Part model, mm, in its own coordinate system. A direction names the side the tool comes from. Coordinates: 2 decimals unless noted, no trailing zeros. Loops run counter-clockwise (first coordinate to the right, second up) from the corner with the lowest first, then second, coordinate; pieces in that order, holes last.
```python
from build123d import *

# Parameters (mm, degrees)
SKETCH1_R           = 7.9375
BOSS_EXTRUDE1_DEPTH = 27.2415
SKETCH2_R           = 2.4765
CUT_EXTRUDE1_DEPTH  = 49.665241675
CUT_EXTRUDE2_DEPTH  = 49.665241675
SKETCH4_R           = 7.9375
CUT_EXTRUDE3_DEPTH  = 41.615884673
FILLET1_R           = 6.35
FILLET2_R           = 3.175
FILLET3_R           = 12.7
FILLET4_R           = 2.54
FILLET5_R           = 2.54


with BuildPart() as part:
    # Sketch1 → Boss-Extrude1 (new, symmetric)
    with BuildSketch(Plane.XY):
        with BuildLine():
            Line((11.25771962, 2.316093955), (14.0335, -11.176))
            Line((14.0335, -11.176), (14.0335, -28.956))
            Line((14.0335, -28.956), (11.2014, -28.956))
            Line((11.2014, -28.956), (11.2014, -15.1638))
            Line((11.2014, -15.1638), (-11.2014, -15.1638))
            Line((-11.2014, -15.1638), (-11.2014, -28.956))
            Line((-11.2014, -28.956), (-14.0335, -28.956))
            Line((-14.0335, -28.956), (-14.0335, -11.176))
            Line((-14.0335, -11.176), (-11.25771962, 2.316093955))
            ThreePointArc((-11.25771962, 2.316093955), (0, 11.4935), (11.25771962, 2.316093955))
        make_face()
        Circle(SKETCH1_R, mode=Mode.SUBTRACT)
    extrude(amount=BOSS_EXTRUDE1_DEPTH, both=True)

    # Sketch2 → Cut-Extrude1 (cut, through all)
    with BuildSketch(Plane(origin=(14.0335, 0, 0), x_dir=(0, 0, -1), z_dir=(1, 0, 0))):
        with Locations(Location((-20.066, -22.7838, 0), (0, 0, 90))):
            Circle(SKETCH2_R)
        with Locations(Location((-12.7, -22.7838, 0), (0, 0, 90))):
            Circle(SKETCH2_R)
        with Locations(Location((-5.334, -22.7838, 0), (0, 0, 90))):
            Circle(SKETCH2_R)
        with Locations(Location((5.334, -22.7838, 0), (0, 0, 90))):
            Circle(SKETCH2_R)
        with Locations(Location((12.7, -22.7838, 0), (0, 0, 90))):
            Circle(SKETCH2_R)
        with Locations(Location((20.066, -22.7838, 0), (0, 0, 90))):
            Circle(SKETCH2_R)
    extrude(amount=-CUT_EXTRUDE1_DEPTH, mode=Mode.SUBTRACT)

    # Sketch3 → Cut-Extrude2 (cut, through all)
    with BuildSketch(Plane(origin=(14.0335, 0, 0), x_dir=(0, 0, -1), z_dir=(1, 0, 0))):
        Polygon((14.7955, -12.573), (-14.7955, -12.573), (-14.7955, -2.413), (-21.6535, 7.38123903), (-21.6535, 11.4935), (21.6535, 11.4935), (21.6535, 7.38123903), (14.7955, -2.413), align=None)
    extrude(amount=-CUT_EXTRUDE2_DEPTH, mode=Mode.SUBTRACT)

    # Sketch4 → Cut-Extrude3 (cut, through all)
    with BuildSketch(Plane.XZ.offset(15.1638)):
        Circle(SKETCH4_R)
    extrude(amount=-CUT_EXTRUDE3_DEPTH, mode=Mode.SUBTRACT)

    # Fillet1
    fillet1_edges = [part.edges().sort_by_distance(p)[0] for p in [
        (12.61745, -28.956, -27.2415),
        (-12.61745, -28.956, -27.2415),
        (-12.61745, -28.956, 27.2415),
        (12.61745, -28.956, 27.2415),
    ]]
    fillet(fillet1_edges, radius=FILLET1_R)

    # Fillet2
    fillet2_edges = [part.edges().sort_by_distance(p)[0] for p in [
        (0, -12.573, 14.7955),
        (0, -12.573, -14.7955),
    ]]
    fillet(fillet2_edges, radius=FILLET2_R)

    # Fillet3
    # the kernel refuses this fillet: 12.7 mm, written as the material it adds along each edge
    with BuildSketch(Plane(origin=(18.820836014, 7.38123903, 21.6535), x_dir=(0, -0.8191520442889931, -0.5735764363510439), z_dir=(-1, 0, 0))) as fillet3_piece_1_section:
        with BuildLine():
            CenterArc((FILLET3_R * 0.315298788879, -FILLET3_R), FILLET3_R, 90, 35)
            Line((-FILLET3_R * 0.258277647472, -FILLET3_R * 0.180847955711), (0, 0))
            Line((0, 0), (FILLET3_R * 0.315298788879, 0))
        make_face()
    fillet3_piece_1 = extrude(amount=25.91246026, mode=Mode.PRIVATE)
    fillet3_piece_1 = fillet3_piece_1 & Plane(origin=(0, 0, 21.359418529), x_dir=(-0.9794857632595162, 0.20151337318382392, 0), z_dir=(0, 0, 1)) * Cylinder(11.4935, 68, mode=Mode.PRIVATE)
    fillet3_piece_1 = fillet3_piece_1 - Plane(origin=(0, 0, 21.359418529), x_dir=(1, 0, 0), z_dir=(0, 0, -1)) * Cylinder(7.9375, 68, mode=Mode.PRIVATE)
    add(fillet3_piece_1)
    with BuildSketch(Plane(origin=(7.091624245, 7.38123903, 21.6535), x_dir=(0, -0.8191520442889934, -0.5735764363510438), z_dir=(-1, 0, 0))) as fillet3_piece_2_section:
        with BuildLine():
            CenterArc((FILLET3_R * 0.315298788879, -FILLET3_R), FILLET3_R, 90, 35)
            Line((-FILLET3_R * 0.258277647472, -FILLET3_R * 0.180847955711), (0, 0))
            Line((0, 0), (FILLET3_R * 0.315298788879, 0))
        make_face()
    fillet3_piece_2 = extrude(amount=25.91246026, mode=Mode.PRIVATE)
    fillet3_piece_2 = fillet3_piece_2 & Plane(origin=(0, 0, 21.359421055), x_dir=(-0.9794857632595162, 0.20151337318382392, 0), z_dir=(0, 0, 1)) * Cylinder(11.4935, 68, mode=Mode.PRIVATE)
    fillet3_piece_2 = fillet3_piece_2 - Plane(origin=(0, 0, 21.359421055), x_dir=(1, 0, 0), z_dir=(0, 0, -1)) * Cylinder(7.9375, 68, mode=Mode.PRIVATE)
    add(fillet3_piece_2)
    with BuildSketch(Plane(origin=(7.091624245, 7.38123903, -21.6535), x_dir=(0, -0.819152044288993, 0.5735764363510443), z_dir=(-1, 0, 0))) as fillet3_piece_3_section:
        with BuildLine():
            CenterArc((FILLET3_R * 0.315298788879, FILLET3_R), FILLET3_R, 235, 35)
            Line((-FILLET3_R * 0.258277647472, FILLET3_R * 0.180847955711), (0, 0))
            Line((0, 0), (FILLET3_R * 0.315298788879, 0))
        make_face()
    fillet3_piece_3 = extrude(amount=25.91246026, mode=Mode.PRIVATE)
    fillet3_piece_3 = fillet3_piece_3 - Plane(origin=(0, 0, -21.359421055), x_dir=(1, 0, 0), z_dir=(0, 0, -1)) * Cylinder(7.9375, 68, mode=Mode.PRIVATE)
    fillet3_piece_3 = fillet3_piece_3 & Plane(origin=(0, 0, -21.359421055), x_dir=(-0.9794857632595162, 0.20151337318382392, 0), z_dir=(0, 0, 1)) * Cylinder(11.4935, 68, mode=Mode.PRIVATE)
    add(fillet3_piece_3)
    with BuildSketch(Plane(origin=(18.820836014, 7.38123903, -21.6535), x_dir=(0, -0.8191520442889931, 0.5735764363510439), z_dir=(-1, 0, 0))) as fillet3_piece_4_section:
        with BuildLine():
            CenterArc((FILLET3_R * 0.315298788879, FILLET3_R), FILLET3_R, 235, 35)
            Line((-FILLET3_R * 0.258277647472, FILLET3_R * 0.180847955711), (0, 0))
            Line((0, 0), (FILLET3_R * 0.315298788879, 0))
        make_face()
    fillet3_piece_4 = extrude(amount=25.91246026, mode=Mode.PRIVATE)
    fillet3_piece_4 = fillet3_piece_4 & Plane(origin=(0, 0, -21.359418529), x_dir=(-0.9794857632595162, 0.20151337318382392, 0), z_dir=(0, 0, 1)) * Cylinder(11.4935, 68, mode=Mode.PRIVATE)
    fillet3_piece_4 = fillet3_piece_4 - Plane(origin=(0, 0, -21.359418529), x_dir=(1, 0, 0), z_dir=(0, 0, -1)) * Cylinder(7.9375, 68, mode=Mode.PRIVATE)
    add(fillet3_piece_4)

    # Fillet4
    fillet4_edges = [part.edges().sort_by_distance(p)[0] for p in [
        (9.89624428, -2.413, -14.7955),
        (-9.89624428, -2.413, -14.7955),
        (-9.89624428, -2.413, 14.7955),
        (9.89624428, -2.413, 14.7955),
    ]]
    fillet(fillet4_edges, radius=FILLET4_R)

    # Fillet5
    fillet5_edges = [part.edges().sort_by_distance(p)[0] for p in [
        (-14.0335, -11.176, 20.746232014),
        (-14.0335, -11.176, -20.746232014),
        (14.0335, -11.176, -20.746232014),
        (14.0335, -11.176, 20.746232014),
    ]]
    fillet(fillet5_edges, radius=FILLET5_R)


solid = part.part
```
Q1. Probe line 1 (Z direction, x = 2.25, y = -8.5); line 2 (Z direction, x = 0, y = -14.45); line 3 (X direction, y = -16, z = 12). List the from-to ranges inside material, lowest first.
Q2. Tool access for faces 1 (the cylindrical face through (-12.6, -23.11, 22.52)), 2 (the flat face through (-9.409, 1.131, 17.277)): list every direction of +Z, -Z, +X, -X, +Y, -Y with a clear straight run to the whole face (end or side of a thin tool).
Q3. Saw through at D-D (z = -12.7). List the corners of the cut face in (x, y), plus the area to 3 significant figures.
Q4. Mould opens along X. For faces 3 (the cylindrical face through (12.6, -27.05, -25.43)), 4 (the flat face through (-11.201, -22, 0)), 5 (the flat face through (11.201, -22, 0)), 6 (the cylindrical face through (0.22, 11.49, 23.75)) say: released by +X, released by -X, zero draft, split by the parting line, or undercut.
Q5. Saw through at A-A (y = -17.5). List the corners of the cut face in (x, z).
Q6. Saw through at C-C (x = 0.75). Count the separate pieces of the cut face and the enclosed holes in it, plus the area to 3 significant figures.
Q7. Saw through at B-B (z = 0). List the corners of the cut face in (x, y), plus the area to 3 significant figures.
Q8. Drop flat-ended pins along their axis: P1, Ø1, axis at x = -4.5, z = -8.5, coming from the -Y side; P2, Ø4.5, axis at y = -22.78, z = 5.33, coming from the -X side; P3, Ø2, axis at x = -2.5, z = 17.5, coming from the +Y side; P4, Ø11.5, axis at x = -2.5, z = -3.5, coming from the +Y side. Give the stop position or say it passes through.
Checked values:
1. line 1: z = -27.24 to -14.8, 14.8 to 27.24
1. line 2: z = -27.24 to -7.94, 7.94 to 27.24
1. line 3: x = -14.03 to -11.2, 11.2 to 14.03
2. face 1: +X, -X
2. face 2: +X, -X, +Y
3. outline: (-14.03, -28.96) - (-11.2, -28.96) - (-11.2, -25.26) - (-14.03, -25.26) - close; (-14.03, -20.31) - (-11.2, -20.31) - (-11.2, -15.16) - (11.2, -15.16) - (11.2, -20.31) - (14.03, -20.31) - (14.03, -12.38) - (-14.03, -12.38) - close; (11.2, -28.96) - (14.03, -28.96) - (14.03, -25.26) - (11.2, -25.26) - close
3. area: 128 mm2
4. face 3: zero draft
4. face 4: undercut
4. face 5: undercut
4. face 6: split by the parting line
5. outline: (-14.03, -27.24) - (-11.2, -27.24) - (-11.2, 27.24) - (-14.03, 27.24) - close; (11.2, -27.24) - (14.03, -27.24) - (14.03, 27.24) - (11.2, 27.24) - close
6. separate pieces: 4
6. enclosed holes: 0
6. area: 262 mm2
7. outline: (-14.03, -28.96) - (-11.2, -28.96) - (-11.2, -15.16) - (-7.94, -15.16) - (-7.94, -12.57) - (-14.03, -12.57) - close; (7.94, -15.16) - (11.2, -15.16) - (11.2, -28.96) - (14.03, -28.96) - (14.03, -12.57) - (7.94, -12.57) - close
7. area: 110 mm2
8. P1: stops at y = -15.16
8. P2: passes through
8. P3: stops at y = -7.12
8. P4: stops at y = -12.57
